Geometry: see drawing. Coordinates: mm, zero at the bounding-box minimum. A direction names the side the tool comes from. Coordinates: 2 decimals unless noted, no trailing zeros. Loops run counter-clockwise (first coordinate to the right, second up) from the corner with the lowest first, then second, coordinate; pieces in that order, holes last. Notation, with made-up numbers: M 11.5,-11.75 L 42.5,-11.75 A19 ccw 42.5,-3.75 Z; hole C 1,85.25 d4. An arc over 180 degrees is marked long. One line per question, with ' | ' between items. Start each with the question number.
1. Ray query, probe 1 along Z at (x, y) = (13.5, 6.5); probe 2 along Y at (x, z) = (7.5, 20); probe 3 along X at (y, z) = (8.75, 16) (1 decimal). Return the intervals inside material, ascending.
2. Pin query (flat end, axial travel): P1, Ø3, axis at y = 7, z = 25, coming from the -X side; P2, Ø5, axis at x = 8, z = 21, coming from the -Y side; P3, Ø5, axis at y = 4, z = 14.5, coming from the -X side; P4, Ø3, axis at y = 2, z = 9.5, coming from the +X side. Return the tip coordinate at first contact, or that it passes through.
3. Section query B-B, the plane y = 7.25. Output: boundary loops of the cut face in (x, z) (1 decimal).
4. Access query for the marked faces 1 and 2. Directions: +Z, -Z, +X, -X, +Y, -Y. A direction counts if a zero-diameter tool reaches every point of the face in a straight line with its end or side. Return the directions, or none.
5. Section query A-A, the plane x = 8.5. Output: boundary loops of the cut face in (y, z), and give its area (3 significant figures).
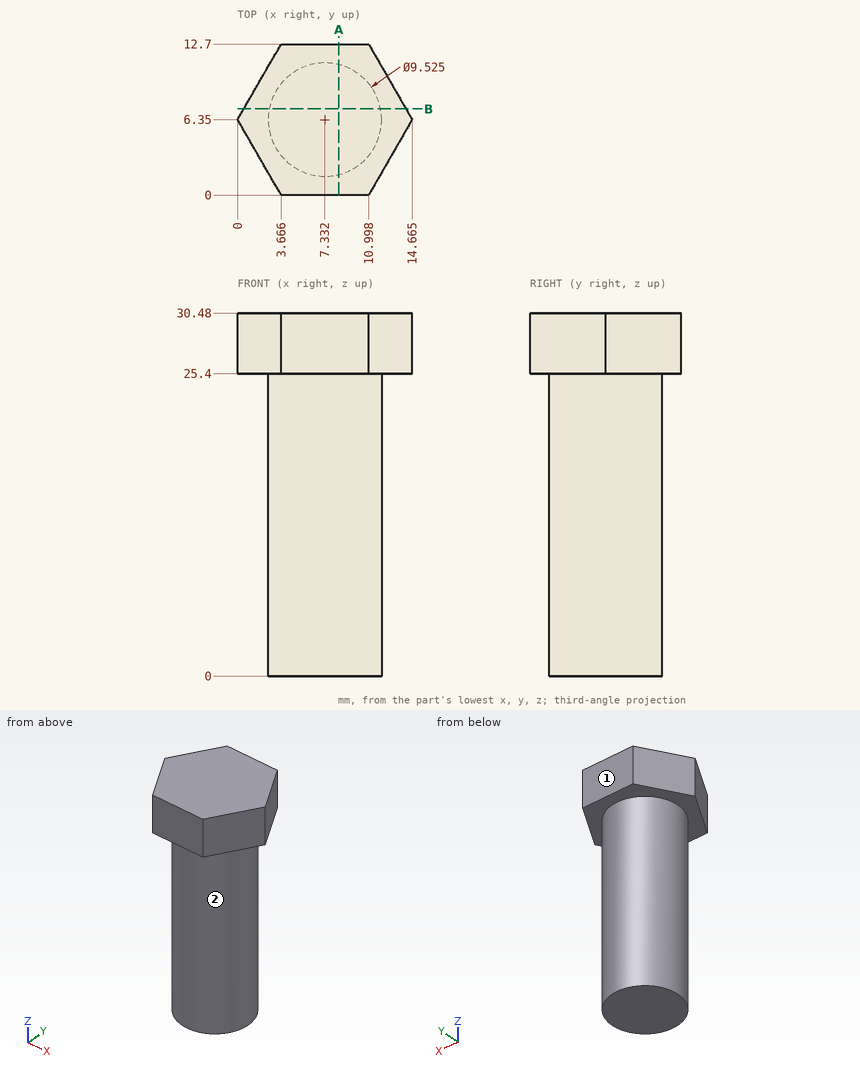
Taken from the geometry:
1) probe 1: 25.4 to 30.48 | probe 2: 1.59 to 11.11 | probe 3: 3.2 to 11.4
2) P1: x = 0 | P2: y = 1.59 | P3: x = 2.57 | P4: x = 11.15
3) outline: M 0.5,25.4 L 2.7,25.4 L 2.7,0 L 12,0 L 12,25.4 L 14.1,25.4 L 14.1,30.5 L 0.5,30.5 Z
4) face 1: +Z, -Z, +X, -X, +Y | face 2: -Z
5) outline: M 0,25.4 L 1.73,25.4 L 1.73,0 L 10.97,0 L 10.97,25.4 L 12.7,25.4 L 12.7,30.48 L 0,30.48 Z | area: 299 mm^2
